from build123d import *

# Parameters (mm, degrees)
SKETCH1_R           = 1.65
SKETCH1_R_2         = 1.5
SKETCH1_R_3         = 1.35
BOSS_EXTRUDE1_DEPTH = 5.842
FILLET1_R           = 18
SKETCH2_R           = 1.5
CUT_EXTRUDE1_DEPTH  = 73.079185373


with BuildPart() as part:
    # Sketch1 → Boss-Extrude1 (new body)
    with BuildSketch(Plane.XY):
        with BuildLine():
            Line((-12.7, 0), (-12.7, 49.186888497))
            ThreePointArc((-12.7, 49.186888497), (0, -50.8), (12.7, 49.186888497))
            Line((12.7, 49.186888497), (12.7, 0))
            ThreePointArc((12.7, 0), (0, -12.7), (-12.7, 0))
        make_face()
        with Locations((22, 0)):
            Circle(SKETCH1_R, mode=Mode.SUBTRACT)
        with Locations((0, -22)):
            Circle(SKETCH1_R, mode=Mode.SUBTRACT)
        with Locations((-22, 0)):
            Circle(SKETCH1_R, mode=Mode.SUBTRACT)
        with Locations((-45.72, 0)):
            Circle(SKETCH1_R_2, mode=Mode.SUBTRACT)
        with Locations((45.72, 0)):
            Circle(SKETCH1_R_2, mode=Mode.SUBTRACT)
        with Locations((0, -45.72)):
            Circle(SKETCH1_R_2, mode=Mode.SUBTRACT)
        with Locations((39.594681461, 22.86)):
            Circle(SKETCH1_R_3, mode=Mode.SUBTRACT)
        with Locations((39.594681461, -22.86)):
            Circle(SKETCH1_R_3, mode=Mode.SUBTRACT)
        with Locations((-39.594681461, -22.86)):
            Circle(SKETCH1_R_3, mode=Mode.SUBTRACT)
        with Locations((-39.594681461, 22.86)):
            Circle(SKETCH1_R_3, mode=Mode.SUBTRACT)
    extrude(amount=BOSS_EXTRUDE1_DEPTH)

    # Fillet1
    fillet1_edges = [part.edges().sort_by_distance(p)[0] for p in [
        (12.7, 49.186888497, 2.921),
        (-12.7, 49.186888497, 2.921),
    ]]
    fillet(fillet1_edges, radius=FILLET1_R)

    # Sketch2 → Cut-Extrude1 (cut, through all)
    with BuildSketch(Plane.XY.offset(5.842)):
        with Locations((-15.556349186, -15.556349186)):
            Circle(SKETCH2_R)
        with Locations((-15.556349186, 15.556349186)):
            Circle(SKETCH2_R)
        with Locations((15.556349186, 15.556349186)):
            Circle(SKETCH2_R)
        with Locations((15.556349186, -15.556349186)):
            Circle(SKETCH2_R)
    extrude(amount=-CUT_EXTRUDE1_DEPTH, mode=Mode.SUBTRACT)


solid = part.part
Read the model definition and answer for the solid it produces. Units are mm, in the model's axes. A direction names the side the tool comes from. Give positions to 0.01 mm unless a question says otherwise; leave off trailing zeros. Write each loop counter-clockwise with the first axis right and the second up, starting at its lowest first coordinate (ties: lowest second). Pieces come first, ordered by that corner, then holes. Notation, with made-up numbers: M 87,66.25 L 141,66.25 A25 ccw 141,84.25 Z; hole C 88.5,-13 d3. An arc over 180 degrees is marked long. One line per item, written item: value. Start each with the question number.
(1) Find section A-A (y = -45.72). Determine the outline of the cut face in (x, z).
(2) Flat-ended cylindrical pins translate along their axes: pin 1 Ø2 at (x, y) = (-22, 0) entering from -Z; pin 2 Ø3 at (y, z) = (-9.5, 1) entering from -X; pin 3 Ø1.8 at (y, z) = (3.5, 3.5) entering from -X; pin 4 Ø1 at (x, z) = (3, 5) entering from -Y. Find the tip coordinate at first contact, or state that the pin passes through.
(3) A tool of negligible diameter and unlimited length cuts with its end or side. For faces 5 (the flat face through (-12.7, 6, 3)), 6 (the cylindrical face through (15.23, -17.02, 2.96)), from which of +Z, -Z, +X, -X, +Y, -Y can it reach the whole face along a straight path? Write none if from no direction.
(4) Find the intervals of material crossed by line 1 (Y direction, x = 0, z = 4.2); line 2 (X direction, y = 6, z = 4.25); line 3 (X direction, y = 7, z = 0.95), in increasing order.
(5) Determine the mould class of faces 1 (the cylindrical face through (-1.37, -50.78, 2.88)), 2 (the flat face through (-1, -19, 0)), 3 (the cylindrical face through (14.45, 16.57, 2.96)), 4 (the cylindrical face through (-40.59, -21.95, 2.88)) for opening direction X: pulls with the +X half, pulls with the -X half, needs draft (parallel to the pull), parting line crosses it, or undercut.
(6) Find section B-B (z = 2.4). Give the number of separate pieces and of enclosed holes in the cut face, plus the area to 3 significant figures.
(7) Find section C-C (x = 45.72). Determine the outline of the cut face in (y, z), plus the area to 3 significant figures.
(8) Find section D-D (x = -28.5). Determine the outline of the cut face in (y, z), plus the area to 3 significant figures.
Results below:
1. outline: M -22.14,0 L -1.5,0 L -1.5,5.84 L -22.14,5.84 Z; M 1.5,0 L 22.14,0 L 22.14,5.84 L 1.5,5.84 Z
2. pin 1: passes through
2. pin 2: stops at x = -50.17
2. pin 3: stops at x = -50.73
2. pin 4: stops at y = -50.74
3. face 5: +Z, -Z, +Y
3. face 6: +Z, -Z
4. line 1: y = -50.8 to -47.22, -44.22 to -23.65, -20.35 to -12.7
4. line 2: x = -50.44 to -12.7, 12.7 to 50.44
4. line 3: x = -50.32 to -12.7, 12.7 to 50.32
5. face 1: parting line crosses it
5. face 2: needs draft
5. face 3: undercut
5. face 4: undercut
6. separate pieces: 1
6. enclosed holes: 14
6. area: 5,590 mm^2
7. outline: M -22.14,0 L -1.5,0 L -1.5,5.84 L -22.14,5.84 Z; M 1.5,0 L 21.47,0 L 21.47,5.84 L 1.5,5.84 Z
7. area: 237 mm^2
8. outline: M -42.05,0 L 29.41,0 L 29.41,5.84 L -42.05,5.84 Z
8. area: 417 mm^2
